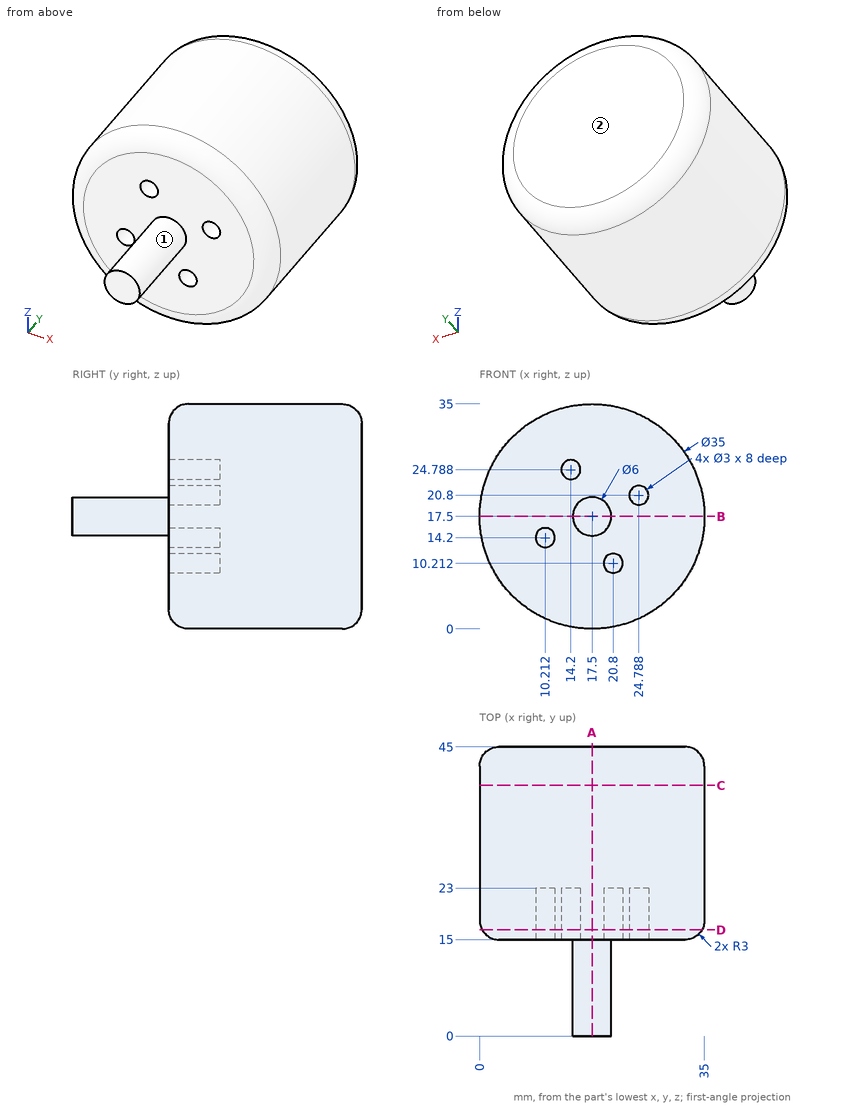
Part print with two shaded views. Sizes in mm from the minimum x, y, z corner. A direction names the side the tool comes from. Round coordinates to 2 decimals unless told otherwise and drop trailing zeros. Order: outer loops, then holes, each group sorted by start corner. A loop starts at its lowest first (then second) coordinate and runs counter-clockwise, first axis right, second up. Notation, with made-up numbers: M 16,-26.5 L 49,-26.5 A27 ccw 49,-8.5 Z; hole C 35,-27 d11. An arc over 180 degrees is marked long. Use CSV: the item, a comma, the result in double quotes. Start each with the question number.
(1) Cut at D-D on y = 16.5. List the corners of the cut face in (x, z), then the cut area to 3 significant figures.
(2) Drill centre lines: probe 1 along Y at (x, z) = (15, 11); probe 2 along Z at (x, y) = (20.5, 18); probe 3 along Z at (x, y) = (20, 16) (1 decimal). Where is each one in solid material? Low to high.
(3) Cut at C-C on y = 39. List the corners of the cut face in (x, z), then the cut area to 3 significant figures.
(4) Flat gauge pins, fed straight in: P1, Ø2.5, axis at x = 10.5, z = 14.5, coming from the -Y side; P2, Ø12, axis at y = 15.5, z = 5, coming from the +X side; P3, Ø12, axis at x = 10.5, y = 36.5, coming from the +Z side. Where does each tip first touch, or does it go through?
(5) Cut at A-A on x = 17.5. List the corners of the cut face in (y, z).
(6) Cut at B-B on z = 17.5. List the corners of the cut face in (x, y).
(7) Tool access for the marked faces 1 and 2: list every direction of +Z, -Z, +X, -X, +Y, -Y with a clear straight run to the whole face (end or side of a thin tool).
Findings:
1,outline,"C 17.5,17.5 d34.2; hole C 10.21,14.2 d3; hole C 14.2,24.79 d3; hole C 20.8,10.21 d3; hole C 24.79,20.8 d3"
1,area,"890 mm^2"
2,probe 1,"y = 15 to 45"
2,probe 2,"z = 0.26 to 8.74, 11.68 to 34.74"
2,probe 3,"z = 1 to 8.9, 11.5 to 34"
3,outline,"C 17.5,17.5 d35"
3,area,"962 mm^2"
4,P1,"stops at y = 15"
4,P2,"stops at x = 33.56"
4,P3,"stops at z = 34.97"
5,outline,"M 0,14.5 L 15,14.5 L 15,3 A3 ccw 18,0 L 42,0 A3 ccw 45,3 L 45,32 A3 ccw 42,35 L 18,35 A3 ccw 15,32 L 15,20.5 L 0,20.5 Z"
6,outline,"M 0,18 A3 ccw 3,15 L 14.5,15 L 14.5,0 L 20.5,0 L 20.5,15 L 32,15 A3 ccw 35,18 L 35,42 A3 ccw 32,45 L 3,45 A3 ccw 0,42 Z"
7,face 1,"-Y"
7,face 2,"+Z, -Z, +X, -X, +Y"
